The model under review builds one solid part; all positions refer to its coordinate system, in mm. Give positions to 0.01 mm unless a question says otherwise; leave off trailing zeros. Loops run counter-clockwise (first coordinate to the right, second up) from the corner with the lowest first, then second, coordinate; pieces in that order, holes last. Notation, with made-up numbers: M 70,67 L 97,67 A31 ccw 97,104 Z; hole C -4,13.5 d8. An arc over 180 degrees is marked long. One line per item, written item: value. Start each with the question number.
Q1. We need section B-B on x = 0. Write out the cut boundary in (y, z), plus the area to 3 significant figures.
Q2. We need section A-A on x = -109.5. Write out the cut boundary in (y, z), plus the area to 3 significant figures.
Q3. For pin 1 (4 mm diameter, centred on x = 14.85, y = 54.5, fed in from +Z), flat-tipped, find the tip position at first contact; note if it passes through.
Q4. We need section C-C on z = -3.1. Give the number of separate pieces and of enclosed holes in the cut face, plus the area to 3 significant figures.
Q5. To check wall thickness, follow line 1 along X through (y, z) = (40, -3.8); line 2 along X through (y, z) = (19, -1.2); line 3 along X through (y, z) = (41, -4.5). State the ranges of each line that lie inside material, in increasing order. Write a range as from..to.
```python
from build123d import *

# Parameters (mm, degrees)
SKETCH1_W          = 788
SKETCH1_H          = 150
BASE_FLANGE1_DEPTH = 6
SKETCH2_R          = 2.25
SKETCH2_R_2        = 17
SKETCH2_W          = 50
SKETCH2_H          = 50
CUT_EXTRUDE1_DEPTH = 402.119682888
SKETCH3_R          = 3.25
CUT_EXTRUDE2_DEPTH = 10


# Sheet-metal steps are written as plain solids
with BuildPart() as part:
    # Sketch1 → Base-Flange1 (new body)
    with BuildSketch(Plane.XY):
        Rectangle(SKETCH1_W, SKETCH1_H)
    extrude(amount=-BASE_FLANGE1_DEPTH)

    # Sketch2 → Cut-Extrude1 (cut, through all)
    with BuildSketch(Plane.XY):
        with Locations((14.849242405, 54.499242405)):
            Circle(SKETCH2_R)
        with Locations((-14.849242405, 54.499242405)):
            Circle(SKETCH2_R)
        with Locations((-14.849242405, 24.800757595)):
            Circle(SKETCH2_R)
        with Locations((14.849242405, 24.800757595)):
            Circle(SKETCH2_R)
        with Locations((0, 39.65)):
            Circle(SKETCH2_R_2)
        with Locations((-125, 30)):
            Rectangle(SKETCH2_W, SKETCH2_H)
        with Locations((125, 30)):
            Rectangle(SKETCH2_W, SKETCH2_H)
    extrude(amount=-CUT_EXTRUDE1_DEPTH, mode=Mode.SUBTRACT)

    # Sketch3 → Cut-Extrude2 (cut)
    with BuildSketch(Plane.XY):
        with Locations((369, -20)):
            Circle(SKETCH3_R)
        with Locations((-369, -20)):
            Circle(SKETCH3_R)
    extrude(amount=-CUT_EXTRUDE2_DEPTH, mode=Mode.SUBTRACT)


solid = part.part
```
Solved:
1. outline: M -75,-6 L 22.65,-6 L 22.65,0 L -75,0 Z; M 56.65,-6 L 75,-6 L 75,0 L 56.65,0 Z
1. area: 696 mm2
2. outline: M -75,-6 L 5,-6 L 5,0 L -75,0 Z; M 55,-6 L 75,-6 L 75,0 L 55,0 Z
2. area: 600 mm2
3. pin 1: through
4. separate pieces: 1
4. enclosed holes: 9
4. area: 112,000 mm2
5. line 1: -394..-150, -100..-17, 17..100, 150..394
5. line 2: -394..-150, -100..100, 150..394
5. line 3: -394..-150, -100..-16.95, 16.95..100, 150..394
